```python
from build123d import *

# Parameters (mm, degrees)
CROQUIS1_W              = 50
CROQUIS1_H              = 110
SALIENTE_EXTRUIR1_DEPTH = 2.5
CROQUIS2_R              = 2.5
SALIENTE_EXTRUIR2_DEPTH = 15
CHAFL_N1_SIZE           = 1.3
REDONDEO1_R             = 1
CORTAR_EXTRUIR1_DEPTH   = 10
CROQUIS5_R              = 8.912982345
SALIENTE_EXTRUIR5_DEPTH = 7
SALIENTE_EXTRUIR6_DEPTH = 6
CROQUIS6_W              = 48
CROQUIS6_H              = 1.766405202
CROQUIS6_H_2            = 2.105673341
SALIENTE_EXTRUIR7_DEPTH = 4


with BuildPart() as part:
    # Croquis1 → Saliente-Extruir1 (new body)
    with BuildSketch(Plane.XY):
        Rectangle(CROQUIS1_W, CROQUIS1_H)
    extrude(amount=SALIENTE_EXTRUIR1_DEPTH)

    # Croquis2 → Saliente-Extruir2 (add)
    with BuildSketch(Plane.XY.offset(2.5)):
        with Locations((-15, 50)):
            Circle(CROQUIS2_R)
        with Locations((-21, 45)):
            Circle(CROQUIS2_R)
        with Locations((-15, 40)):
            Circle(CROQUIS2_R)
        with Locations((-9, 45)):
            Circle(CROQUIS2_R)
        with Locations((-15, -40)):
            Circle(CROQUIS2_R)
        with Locations((-9, -45)):
            Circle(CROQUIS2_R)
        with Locations((-15, -50)):
            Circle(CROQUIS2_R)
        with Locations((-21, -45)):
            Circle(CROQUIS2_R)
        with Locations(Location((21, -45, 0), (0, 0, 180))):
            Circle(CROQUIS2_R)
        with Locations(Location((15, -50, 0), (0, 0, 180))):
            Circle(CROQUIS2_R)
        with Locations(Location((9, -45, 0), (0, 0, 180))):
            Circle(CROQUIS2_R)
        with Locations(Location((15, -40, 0), (0, 0, 180))):
            Circle(CROQUIS2_R)
        with Locations(Location((21, 45, 0), (0, 0, 180))):
            Circle(CROQUIS2_R)
        with Locations(Location((15, 50, 0), (0, 0, 180))):
            Circle(CROQUIS2_R)
        with Locations(Location((9, 45, 0), (0, 0, 180))):
            Circle(CROQUIS2_R)
        with Locations(Location((15, 40, 0), (0, 0, 180))):
            Circle(CROQUIS2_R)
    extrude(amount=SALIENTE_EXTRUIR2_DEPTH)

    # Chafl_n1
    chafl_n1_edges = [part.edges().sort_by_distance(p)[0] for p in [
        (-17.5, 50, 17.5),
        (-23.5, 45, 17.5),
        (-17.5, 40, 17.5),
        (-11.5, 45, 17.5),
        (-17.5, -40, 17.5),
        (-11.5, -45, 17.5),
        (-17.5, -50, 17.5),
        (-23.5, -45, 17.5),
        (23.5, -45, 17.5),
        (17.5, -50, 17.5),
        (11.5, -45, 17.5),
        (17.5, -40, 17.5),
        (23.5, 45, 17.5),
        (17.5, 50, 17.5),
        (11.5, 45, 17.5),
        (17.5, 40, 17.5),
    ]]
    chamfer(chafl_n1_edges, length=CHAFL_N1_SIZE)

    # Redondeo1
    redondeo1_edges = [part.edges().sort_by_distance(p)[0] for p in [
        (0, -55, 0),
        (-25, 0, 0),
        (0, 55, 0),
        (25, 0, 0),
    ]]
    fillet(redondeo1_edges, radius=REDONDEO1_R)

    # Croquis3 → Cortar-Extruir1 (cut)
    with BuildSketch(Plane(origin=(0, 0, 0), x_dir=(-1, 0, 0), z_dir=(0, 0, -1))):
        with BuildLine():
            add(Edge.make_bspline(
                [(22.361475253, -39.186991388), (10.271319675, 11.528482347), (23.288602916, 40.714890738)],
                knots=[0, 0, 0, 1, 1, 1], degree=2))
            add(Edge.make_bspline(
                [(22.361475253, -39.186991388), (20.200722134, -14.449114626), (20.113642926, 12.226208442), (23.288602916, 40.714890738)],
                knots=[0, 0, 0, 0, 1, 1, 1, 1], degree=3))
        make_face()
        with BuildLine():
            add(Edge.make_bspline(
                [(-22.361475253, -39.186991388), (-20.200722134, -14.449114626), (-20.113642926, 12.226208442), (-23.288602916, 40.714890738)],
                knots=[0, 0, 0, 0, 1, 1, 1, 1], degree=3))
            add(Edge.make_bspline(
                [(-22.361475253, -39.186991388), (-10.271319675, 11.528482347), (-23.288602916, 40.714890738)],
                knots=[0, 0, 0, 1, 1, 1], degree=2))
        make_face()
    extrude(amount=-CORTAR_EXTRUIR1_DEPTH, mode=Mode.SUBTRACT)

    # Croquis5 → Saliente-Extruir5 (add)
    with BuildSketch(Plane.XY.offset(2.5)):
        with Locations((-15, 44.758672209)):
            Circle(CROQUIS5_R)
        with Locations(Location((-15, -44.758672209, 0), (0, 0, 180))):
            Circle(CROQUIS5_R)
        with Locations(Location((15, 44.758672209, 0), (0, 0, 180))):
            Circle(CROQUIS5_R)
        with Locations((15, -44.758672209)):
            Circle(CROQUIS5_R)
    extrude(amount=SALIENTE_EXTRUIR5_DEPTH)

    # Croquis4 → Saliente-Extruir6 (add)
    with BuildSketch(Plane(origin=(0, 0, 0), x_dir=(-1, 0, 0), z_dir=(0, 0, -1))):
        Polygon((6.163131116, 11.924666471), (6.163131116, 10.6), (8, 10.6), (8, 9.070517568), (9.349963895, 9.070517568), (9.349963895, 11.924666471), align=None)
        Polygon((-6.163131116, 11.924666471), (-6.163131116, 10.6), (-7.7, 10.6), (-7.7, 9.070517568), (-8.979725427, 9.070517568), (-8.979725427, 11.924666471), align=None)
        Polygon((-7.7, -8.470517568), (-7.7, -10), (-6.163131116, -10), (-6.163131116, -11.324666471), (-8.979725427, -11.324666471), (-8.979725427, -8.470517568), align=None)
        Polygon((8, -8.470517568), (9.349963895, -8.470517568), (9.349963895, -11.324666471), (6.163131116, -11.324666471), (6.163131116, -10), (8, -10), align=None)
    extrude(amount=-SALIENTE_EXTRUIR6_DEPTH)

    # Croquis6 → Saliente-Extruir7 (add)
    with BuildSketch(Plane(origin=(0, 0, 0), x_dir=(-1, 0, 0), z_dir=(0, 0, -1))):
        with Locations((0, 51.133202601)):
            Rectangle(CROQUIS6_W, CROQUIS6_H)
        with Locations((0, -51.002836671)):
            Rectangle(CROQUIS6_W, CROQUIS6_H_2)
    extrude(amount=SALIENTE_EXTRUIR7_DEPTH)


solid = part.part
```
Read the model definition and answer for the solid it produces. Units are mm, in the model's axes. A direction names the side the tool comes from. Give positions to 0.01 mm unless a question says otherwise; leave off trailing zeros. Write each loop counter-clockwise with the first axis right and the second up, starting at its lowest first coordinate (ties: lowest second). Pieces come first, ordered by that corner, then holes. Notation, with made-up numbers: (-37.5, 45) -> (2.5, 45) arc R26 ccw to (2.5, 66) -> close; hole circle Ø2 at (47.25, 77.5). An arc over 180 degrees is marked (long way). Answer as a JSON object with one key per item and string values.
1) A tool of negligible diameter and unlimited length cuts with its end or side. For faces 5 (the flat face through (8.98, -10, 4)), 6 (the flat face through (21, -45, 17.5)), 7 (the flat face through (-8, 11, 6)), 8 (the cylindrical face through (-23, 43.5, 12.8)), from which of +Z, -Z, +X, -X, +Y, -Y can it reach the whole face along a straight path? Write none if from no direction.
Findings below:
{"face 5": "+Z, +X", "face 6": "+Z, +X, -X, +Y, -Y", "face 7": "+Z, +X, -X", "face 8": "+Z"}
2) Section A-A on x = 3.5 is taken. Write down the section's boundary in (y, z).
Findings below:
{"outline": "(-55, 1) arc R1 ccw to (-54, 0) -> (-52.06, 0) -> (-52.06, -4) -> (-49.95, -4) -> (-49.95, 0) -> (50.25, 0) -> (50.25, -4) -> (52.02, -4) -> (52.02, 0) -> (54, 0) arc R1 ccw to (55, 1) -> (55, 2.5) -> (-55, 2.5) -> close"}
3) Section C-C on y = 0.5 is taken. Count the separate pieces of the cut face and the enclosed holes in it, then the cut area to 3 significant figures.
Findings below:
{"separate pieces": "3", "enclosed holes": "0", "area": "103 mm^2"}
4) Section B-B on z = 5 is taken. Write down the section's boundary in (x, y), then the cut area to 3 significant figures.
Findings below:
{"outline": "circle Ø17.83 at (-15, -44.76); circle Ø17.83 at (-15, 44.76); (-9.35, -11.32) -> (-6.16, -11.32) -> (-6.16, -10) -> (-8, -10) -> (-8, -8.47) -> (-9.35, -8.47) -> close; (-9.35, 9.07) -> (-8, 9.07) -> (-8, 10.6) -> (-6.16, 10.6) -> (-6.16, 11.92) -> (-9.35, 11.92) -> close; circle Ø17.83 at (15, -44.76); circle Ø17.83 at (15, 44.76); (6.16, -11.32) -> (8.98, -11.32) -> (8.98, -8.47) -> (7.7, -8.47) -> (7.7, -10) -> (6.16, -10) -> close; (6.16, 10.6) -> (7.7, 10.6) -> (7.7, 9.07) -> (8.98, 9.07) -> (8.98, 11.92) -> (6.16, 11.92) -> close", "area": "1,020 mm^2"}
5) For a pull along Y with two mould halves and no side action, classify faces 1 (the flat face through (15, 40, 17.5)), 2 (the flat face through (0, 52.016, -2)), 3 (the cylindrical face through (10.887, 52.666, 5.951)), 4 (the cylindrical face through (9.54, 47.44, 12.8)) as pulls with the +Y half, pulls with the -Y half, needs draft (parallel to the pull), parting line crosses it, or undercut.
Findings below:
{"face 1": "needs draft", "face 2": "pulls with the +Y half", "face 3": "undercut", "face 4": "undercut"}
6) Straight lines are drawn through the part: probe 1 along Y at (x, z) = (15, 16); probe 2 along Y at (x, z) = (16.5, 12.75); probe 3 along Y at (x, z) = (-19.5, -2.25). For each, find the intervals that lie inside material, in ascending order. Write a range as from..to.
Findings below:
{"probe 1": "y = -52.5..-47.5, -42.5..-37.5, 37.5..42.5, 47.5..52.5", "probe 2": "y = -52..-48, -42..-38, 38..42, 48..52", "probe 3": "y = -52.06..-49.95, 50.25..52.02"}
7) Flat-ended cylindrical pins translate along their axes: pin 1 Ø2.5 at (y, z) = (-9.5, 4.5) entering from +X; pin 2 Ø1.2 at (x, z) = (6.5, 4.5) entering from -Y; pin 3 Ø2.5 at (y, z) = (-10, 3.5) entering from -X; pin 4 Ø5 at (x, z) = (10.5, 7) entering from -Y. Find the tip coordinate at first contact, or state that the pin passes through.
Findings below:
{"pin 1": "stops at x = 8.98", "pin 2": "stops at y = -48.89", "pin 3": "stops at x = -25", "pin 4": "stops at y = -53.44"}
